The model under review builds one solid part; all positions refer to its coordinate system, in mm. A direction names the side the tool comes from. Coordinates: 2 decimals unless noted, no trailing zeros. Write each loop counter-clockwise with the first axis right and the second up, starting at its lowest first coordinate (ties: lowest second). Pieces come first, ordered by that corner, then holes. Notation, with made-up numbers: (-25, 78.5) - (23, 78.5) arc R37 ccw to (23, 115.5) - close; hole circle Ø9 at (46, 23.25). An arc over 180 degrees is marked (long way). Return JSON: item names as keys, results as strings. Group by question number.
(1) Tool access review of faces 1 (the face through (2, 27, 0)), 2 (the face through (0, -25, 0)), 3 (the face through (0.54, -0.35, 2.44)), 4 (the face through (-1, 28, 0)), 5 (the face through (-0.867, 25.986, -3.905)): name each direction out of +Z, -Z, +X, -X, +Y, -Y from which nothing blocks a thin tool from reaching the whole face with its end or side.
(2) To check wall thickness, follow L1, parallel to Y at x = 1.75, z = -1; L2, parallel to Y at x = 2.25, z = 2.5; L3, parallel to Z at x = 0, y = -12. State the ranges of each line that lie inside material, in increasing order. Write a range as from..to.
(3) We need section A-A on y = 24.5. State the section outline as (x, z) points.
(4) We need section B-B on x = 2. State the section outline as (y, z) points.
(5) For pin 1 Ø3.5 at (x, z) = (-3, 1.5) entering from +Y; pin 2 Ø4 at (x, z) = (1, 3) entering from +Y; pin 3 Ø3 at (y, z) = (21, 0) entering from +X, all flat-tipped, find the tip position at first contact; note any pin that passes through.
(6) We need section C-C on x = -1.75. State the section outline as (y, z) points, then the cut area to 3 significant figures.
Autodesk Inventor part; units mm, degrees
ref_plane "YZ Plane" through (0, 0, 0) normal (1, 0, 0) x (0, 1, 0)
ref_plane "XZ Plane" through (0, 0, 0) normal (0, 1, 0) x (-1, 0, 0)
ref_plane "XY Plane" through (0, 0, 0) normal (0, 0, 1) x (1, 0, 0)
sketch "Sketch1" plane through (0, 0, 0) normal (0, 1, 0) x (-1, 0, 0)
  circle A0 centre (0, 0) radius 2.5
  dimension "d0" = 5
extrude "Extrusion1" add sketch "Sketch1" along normal mid plane 50
sketch "Sketch9" plane through (0, 25, 0) normal (0, 1, 0) x (1, 0, 0)
  circle A0 centre (0, 0) radius 4
  dimension "d56" = 8
extrude "Extrusion2" add sketch "Sketch9" along normal blind 2
sketch "Sketch10" plane through (0, 0, 0) normal (1, 0, 0) x (0, 1, 0)
  line L0 (27, 4) -> (30, 4)
  line L1 (30, 4) -> (30, -4)
  line L2 (30, -4) -> (27, -4)
  line L3 (27, -4) -> (27, 4)
  line L4 (27, -4) -> (27, 4)
  point P0 (0, 0)
  point P1 (27, 0)
  point P2 (30, 0)
  dimension "d59" = 8
  dimension "d60" = 3
extrude "Extrusion3" add sketch "Sketch10" along normal mid plane 2
sketch "Sketch11" plane through (0, 0, 0) normal (1, 0, 0) x (0, 1, 0)
  line L0 (32, 0) -> (32, -5)
  line L1 (27, -4) -> (27, -5)
  line L2 (27, -5) -> (32, -5)
  line L3 (30, 4) -> (30, -4)
  line L4 (32, 0) -> (30, 0)
  line L5 (-36.2, 0) -> (42.2, 0)
  line L6 (30, -4) -> (27, -4)
  arc A0 (27, -4) -> (30, 0) centre (25.8333, 0) ccw
  point P0 (0, 0)
  point P1 (27, 4)
  point P2 (31, 0)
  point P3 (27, -3.873)
  dimension "d65" = 5
  dimension "d68" = 2
revolve "Revolution5" cut sketch "Sketch11" angle 360 about axis through (0, -10, 0) along (0, 1, 0)
thread "Thread4"
equation "\"d23\" = 55deg"
equation "\"Sketch3_Pitch\" = 0.8"
equation "\"d44\" = 55deg"
equation "\"Sketch6_Pitch\" = 1.27"
properties part number "LeadScrew"
Ans:
{
 "1": {"face 1": "+Z, -Z, +X, +Y", "face 2": "+Z, -Z, +X, -X, -Y", "face 3": "-Y", "face 4": "+Z, -Z, -X, +Y", "face 5": "+Y, -Y"},
 "2": {"L1": "-25..27", "L2": "25..27", "L3": "-2.5..2.5"},
 "3": {"outline": "circle Ø5 at (0, 0)"},
 "4": {"outline": "(-25, -1.5) - (25, -1.5) - (25, -3.46) - (27, -3.46) - (27, 3.46) - (25, 3.46) - (25, 1.5) - (-25, 1.5) - close"},
 "5": {"pin 1": "y = 27", "pin 2": "y = 29.83", "pin 3": "x = 2.5"},
 "6": {"outline": "(-25, -1.79) - (25, -1.79) - (25, -3.6) - (27, -3.6) - (27, 3.6) - (25, 3.6) - (25, 1.79) - (-25, 1.79) - close", "area": "193 mm²"}
}
